Autodesk Fusion 360 part; units mm, degrees
sketch "Sketch2" plane through (0, 0, 0) normal (0, 1, 0) x (1, 0, 0)
  circle A0 centre (0, 0) radius 24
  circle A1 centre (0, 0) radius 25.25
  circle A2 centre (0, 0) radius 27
  dimension "d6" = 48
  dimension "d29" = 50.5
  dimension "d37" = 54
extrude "Extrude1" add sketch "Sketch2" along normal blind 31 contours A2
sketch "Sketch3" plane through (0, 0, 0) normal (1, 0, 0) x (0, 0, -1)
  ellipse E0 centre (0, 14.5) end of major axis (-6.75, 14.5) minor radius 4.5
  line L0 (6.75, 14.5) -> (-6.75, 14.5)
  line L1 (0, 19) -> (0, 10)
  dimension "d18" = 13.5
  dimension "d20" = 14.5
  dimension "d49" = 4.5
extrude "Extrude8" cut sketch "Sketch3" along normal mid plane 60
ref_plane "WorkPlane3" through (0, 27.5, 0) normal (0, -1, 0) x (-1, 0, 0)
ref_plane "WorkPlane4" through (0, 52.5, 0) normal (0, -1, 0) x (-1, 0, 0)
sketch "Sketch7" plane through (0, 52.5, 0) normal (0, -1, 0) x (1, 0, 0)
  circle A0 centre (0, 0) radius 23
  circle A1 centre (0, 0) radius 24.5
  dimension "d63" = 46
  dimension "d64" = 49
sketch "Sketch8" plane through (0, 27.5, 0) normal (0, -1, 0) x (1, 0, 0)
  circle A0 centre (0, 0) radius 25
  circle A1 centre (0, 0) radius 23.5
  circle A2 centre (0, 0) radius 27
  dimension "d67" = 50
  dimension "d68" = 47
  dimension "d76" = 54
ref_plane "WorkPlane5" through (0, 42.5, 0) normal (0, -1, 0) x (1, 0, 0)
sketch "Sketch10" plane through (0, 42.5, 0) normal (0, -1, 0) x (1, 0, 0)
  circle A0 centre (0, 0) radius 23.5
  circle A1 centre (0, 0) radius 25
  dimension "d70" = 47
  dimension "d71" = 50
extrude "Extrude14" add sketch "Sketch8" against normal blind 3.5 contours A0 | A2
extrude "Extrude13" add sketch "Sketch8" against normal blind 15 contours A0
loft "Loft1" add profiles "Sketch10", "Sketch7" section 1 section 2
loft "Loft2" cut profiles "Sketch7", "Sketch10" section 1 contours A0 section 2 contours A0
chamfer "Chamfer5" distance 2 angle 45 1 edges at (-23.3082, 31, -9.0404)
chamfer "Chamfer6" distance 1.75 angle 45 1 edges at (-23.5413, 27.5, 9.1308)
Verification items for the finished model (mm, model axes). A direction names the side the tool comes from. Coordinates: 2 decimals unless noted, no trailing zeros. Order: outer loops, then holes, each group sorted by start corner. A loop starts at its lowest first (then second) coordinate and runs counter-clockwise, first axis right, second up. Notation, with made-up numbers: (-10, 48) -> (23, 48) arc R24 ccw to (23, 79) -> close; hole circle Ø8 at (28, 11). An arc over 180 degrees is marked (long way). Put each result on its own line as item: value. Start each with the question number.
1. Cross-section at B-B, the plane y = 7. Record the boundary of the cut face in (x, z), then the cut area to 3 significant figures.
2. Go/stop test with flat-tipped pins: pin 1 Ø2 at (y, z) = (42, -13) entering from -X; pin 2 Ø4 at (y, z) = (21, 4) entering from -X; pin 3 Ø1.5 at (x, y) = (4.5, 17.5) entering from -Z. Record where each tip stops, or that it passes through.
3. Cross-section at C-C, the plane z = 2. Count the separate pieces of the cut face and the enclosed holes in it, then the cut area to 3 significant figures.
4. Access from +Z, -Z, +X, -X, +Y, -Y to the whole of each face (thin tool, end or side, straight path). Record for faces 1 (the flat face through (18, 0, 18)), 2 (the cylindrical face through (24.084, 12.695, 7.584)), 3 (the cylindrical face through (23.846, 37.683, 7.509)).
5. Cross-section at D-D, the plane y = 40. Record the boundary of the cut face in (x, z).
6. Material ranges on L1, parallel to X at y = 9, z = 0; L2, parallel to X at y = 35, z = -7, recorded low to high. Write a range as [from, to].
Computed:
1. outline: circle Ø54 at (0, 0); hole circle Ø50.5 at (0, 0)
1. area: 287 mm2
2. pin 1: x = -21.93
2. pin 2: x = -26.93
2. pin 3: z = -26.74
3. separate pieces: 4
3. enclosed holes: 0
3. area: 163 mm2
4. face 1: +Z, -Z, +X, -X, -Y
4. face 2: -Y
4. face 3: +Y
5. outline: circle Ø50 at (0, 0); hole circle Ø47 at (0, 0)
6. L1: [-27, -25.25], [25.25, 27]
6. L2: [-24, -22.43], [22.43, 24]
